Input: part model. Units: mm. Frame: model coordinates. A direction names the side the tool comes from. Coordinates: 2 decimals unless noted, no trailing zeros. Loops run counter-clockwise (first coordinate to the right, second up) from the corner with the lowest first, then second, coordinate; pieces in that order, holes last. Notation, with made-up numbers: (26.5, 51.25) -> (34.5, 51.25) arc R12 cw to (34.5, 66.25) -> close; hole circle Ø4 at (-27.5, 44). An arc over 180 degrees is marked (long way). Answer as a JSON object with one key per item and string values.
Autodesk Inventor part; units mm, degrees
ref_plane "YZ Plane" through (0, 0, 0) normal (1, 0, 0) x (0, 1, 0)
ref_plane "XZ Plane" through (0, 0, 0) normal (0, 1, 0) x (-1, 0, 0)
ref_plane "XY Plane" through (0, 0, 0) normal (0, 0, 1) x (1, 0, 0)
sketch "Sketch1" plane through (0, 0, 0) normal (0, 0, 1) x (1, 0, 0)
  line L0 (-8.8422, 6.5161) -> (13.7638, 6.5161)
  line L1 (13.7638, -16.0899) -> (-8.8422, -16.0899)
  circle A0 centre (2.4608, -4.7869) radius 4.8768
  arc A1 (-8.8422, -9.6637) -> (-8.8422, 0.0899) centre (-8.8422, -4.7869) ccw
  line L2 (-8.8422, -16.0899) -> (-8.8422, -9.6637)
  line L3 (-8.8422, 0.0899) -> (-8.8422, 6.5161)
  arc A2 (13.7638, 0.0899) -> (13.7638, -9.6637) centre (13.7638, -4.7869) ccw
  line L4 (13.7638, 6.5161) -> (13.7638, 0.0899)
  line L5 (13.7638, -9.6637) -> (13.7638, -16.0899)
  dimension "d2" = 22.606
  dimension "d3" = 22.606
  dimension "d4" = 9.7536
  dimension "d5" = 9.7536
extrude "Extrusion1" add sketch "Sketch1" along normal blind 1.397
fillet "Fillet1" radius 3.175 4 edges at (-8.8422, 6.5161, 0.6985) (13.7638, 6.5161, 0.6985) (13.7638, -16.0899, 0.6985) (-8.8422, -16.0899, 0.6985)
sketch "Sketch2" plane through (0, 0, 1.397) normal (0, 0, 1) x (1, 0, 0)
  line L0 (-8.8422, 3.3411) -> (-8.8422, 0.0899)
  circle A0 centre (-6.5606, 4.3162) radius 1.397
  line L1 (10.5888, 6.5161) -> (-5.6672, 6.5161)
  arc A1 (-8.8422, -9.6637) -> (-8.8422, 0.0899) centre (-8.8422, -4.7869) ccw
  arc A2 (13.7638, 0.0899) -> (13.7638, -9.6637) centre (13.7638, -4.7869) ccw
  circle A3 centre (-6.5606, -13.89) radius 1.397
  line L2 (-5.6672, -16.0899) -> (10.5888, -16.0899)
  circle A4 centre (11.4822, 4.3162) radius 1.397
  circle A5 centre (11.4822, -13.89) radius 1.397
  point P0 (0, 0)
  dimension "d9" = 2.794
extrude "Extrusion2" cut sketch "Sketch2" against normal blind 1.397
sketch "Sketch3" plane through (0, 0, 1.397) normal (0, 0, 1) x (1, 0, 0)
  line L0 (2.4608, -16.0899) -> (2.4608, -9.6637)
  circle A0 centre (2.4608, -4.7869) radius 4.8768
  line L1 (2.4608, -16.0899) -> (0.1367, -16.0899)
  line L2 (-3.0383, -16.0899) -> (7.9599, -16.0899)
  line L3 (2.4608, -16.0899) -> (7.9599, -16.0899)
  line L4 (2.4608, -16.0899) -> (7.9599, -16.0899)
  line L5 (10.5888, -16.0899) -> (-5.6672, -16.0899)
  line L6 (7.9599, -17.9949) -> (7.9599, -16.0899)
  line L7 (-3.0383, -17.9949) -> (-3.0383, -16.0899)
  line L8 (-3.0383, -17.9949) -> (-3.0383, -19.8999)
  line L9 (-3.0383, -19.8999) -> (7.9599, -19.8999)
  line L10 (7.9599, -19.8999) -> (7.9599, -17.9949)
  point P0 (0, 0)
  point P1 (-5.6672, -16.0899)
  dimension "d12" = 5.4991
  dimension "d13" = 5.4991
  dimension "d14" = 1.905
  dimension "d16" = 1.905
extrude "Extrusion3" add sketch "Sketch3" against normal blind 1.397 contours L2 L6 L10 L9 L8 L7 L1
fillet "Fillet2" radius 1.27 2 edges at (7.9599, -16.0899, 0.6985) (-3.0383, -16.0899, 0.6985)
sketch "Sketch4" plane through (-3.0383, -19.8999, 1.397) normal (0, -1, 0) x (1, 0, 0)
  line L0 (10.9982, -1.397) -> (0, -1.397)
  line L1 (10.9982, -1.397) -> (10.9982, -3.4544)
  line L2 (10.9982, -3.4544) -> (0, -3.4544)
  line L3 (0, -3.4544) -> (0, -1.397)
  point P0 (3.0383, -1.397)
  dimension "d20" = 2.0574
extrude "Extrusion4" add sketch "Sketch4" along normal blind 1.397
sketch "Sketch5" plane through (-3.0383, -19.8999, 1.397) normal (0, 1, 0) x (1, 0, 0)
  line L0 (10.9982, 3.4544) -> (10.9982, 1.397)
  line L1 (10.9982, 3.4544) -> (-5.5499, 3.4544)
  line L2 (-5.5499, 3.4544) -> (-5.5499, 14.4526)
  line L3 (-5.5499, 14.4526) -> (16.4973, 14.4526)
  line L4 (10.9982, 1.397) -> (0, 1.397)
  line L5 (0, 3.4544) -> (10.9982, 3.4544)
  line L6 (0, 3.4544) -> (10.9982, 3.4544)
  line L7 (16.4973, 14.4526) -> (16.4973, 3.4544)
  line L8 (16.4973, 3.4544) -> (10.9982, 3.4544)
  point P0 (5.4991, 3.4544)
  point P1 (5.4991, 3.4544)
  dimension "d25" = 22.0472
  dimension "d38" = 10.9982
extrude "Extrusion5" add sketch "Sketch5" against normal blind 1.397
fillet "Fillet3" radius 1.27 2 edges at (-3.0383, -20.5984, -2.0574) (7.9599, -20.5984, -2.0574)
fillet "Fillet4" radius 0.508 4 edges at (-8.5882, -20.5984, -2.0574) (-8.5882, -20.5984, -13.0556) (13.459, -20.5984, -2.0574) (13.459, -20.5984, -13.0556)
sketch "Sketch8" plane through (-3.0383, -19.8999, 0) normal (0, 0, 1) x (1, 0, 0)
  line L0 (0, 0) -> (0, -1.397)
  line L1 (0, -1.397) -> (0, 0)
  line L2 (10.9982, 0) -> (10.9982, -1.397)
  line L3 (0, 0) -> (10.9982, 0)
  line L4 (10.9982, 0) -> (10.9982, -1.397)
  line L5 (10.9982, -1.397) -> (0, -1.397)
  point P0 (3.0383, 19.8999)
extrude "Extrusion8" add sketch "Sketch8" along normal blind 1.397
fillet "Fillet5" radius 1.524 1 edges at (2.4608, -21.2969, 1.397)
sketch "Sketch11" plane through (-3.0383, -19.8999, 1.397) normal (0, 1, 0) x (1, 0, 0)
  line L0 (-5.0419, 14.4526) -> (15.9893, 14.4526)
  line L1 (-2.6289, 1.397) -> (13.6271, 1.397)
  line L2 (16.4973, 13.9446) -> (16.4973, 3.9624)
  line L3 (-5.5499, 13.9446) -> (-5.5499, 3.9624)
  circle A0 centre (13.6271, 11.5283) radius 1.5113
  line L4 (6.7183, 3.3528) -> (6.7183, 11.811)
  line L5 (4.2291, 11.811) -> (4.2291, 3.3528)
  arc A1 (4.2291, 3.3528) -> (6.7183, 3.3528) centre (5.4737, 3.3528) ccw
  arc A2 (6.7183, 11.811) -> (4.2291, 11.811) centre (5.4737, 11.811) ccw
  circle A3 centre (13.6271, 6.3787) radius 1.5113
  line L6 (0, 1.524) -> (10.9982, 1.524)
  circle A4 centre (-2.6681, 11.4963) radius 1.5113
  circle A5 centre (-2.6479, 6.3467) radius 1.5113
  point P0 (5.4737, 7.5819)
  dimension "d43" = 3.0226
  dimension "d47" = 2.8702
  dimension "d50" = 2.6416
  dimension "d51" = 1.9558
extrude "Extrusion10" cut sketch "Sketch11" against normal through all
properties part number "mcdave_mount"
1. Mould query, pull axis Y, two halves, no side actions, for faces 1 (the face through (12.86, 5.56, 0.71)), 2 (the face through (5.08, -8.9, 0.69)), 3 (the face through (-6, -21, -2.057)). Classes: pulls with the +Y half, pulls with the -Y half, needs draft (parallel to the pull), parting line crosses it, or undercut.
Reply:
{"face 1": "pulls with the +Y half", "face 2": "undercut", "face 3": "needs draft"}
2. Section query A-A (z = -8.25). Return loops of the section in (x, y), plus the area to 3 significant figures.
Reply:
{"outline": "(-8.59, -21.3) -> (1.19, -21.3) -> (1.19, -19.9) -> (-8.59, -19.9) -> close; (3.68, -21.3) -> (13.46, -21.3) -> (13.46, -19.9) -> (3.68, -19.9) -> close", "area": "27.3 mm2"}
3. Section query C-C (y = -5.25). Return loops of the section in (x, z).
Reply:
{"outline": "(-3.99, 0) -> (-2.39, 0) -> (-2.39, 1.4) -> (-3.99, 1.4) -> close; (7.32, 0) -> (8.91, 0) -> (8.91, 1.4) -> (7.32, 1.4) -> close"}
4. Section query D-D (x = 11). Return loops of the section in (y, z), plus the area to 3 significant figures.
Reply:
{"outline": "(-21.3, -13.06) -> (-19.9, -13.06) -> (-19.9, -11.59) -> (-21.3, -11.59) -> close; (-21.3, -8.68) -> (-19.9, -8.68) -> (-19.9, -6.44) -> (-21.3, -6.44) -> close; (-21.3, -3.53) -> (-19.9, -3.53) -> (-19.9, -2.06) -> (-21.3, -2.06) -> close; (-16.06, 0) -> (-15.2, 0) -> (-15.2, 1.4) -> (-16.06, 1.4) -> close; (-12.58, 0) -> (-8.8, 0) -> (-8.8, 1.4) -> (-12.58, 1.4) -> close; (-0.77, 0) -> (3.01, 0) -> (3.01, 1.4) -> (-0.77, 1.4) -> close; (5.63, 0) -> (6.49, 0) -> (6.49, 1.4) -> (5.63, 1.4) -> close", "area": "20.2 mm2"}
5. Line query: line 1 along Z through (x, y) = (1.5, -12); line 2 along Y through (x, z) = (9.25, -11.25); line 3 along Y through (x, z) = (5.25, 0.25). Output: solid intervals per line, ascending.
Reply:
{"line 1": "z = 0 to 1.4", "line 2": "y = -21.3 to -19.9", "line 3": "y = -21.25 to -8.79, -0.79 to 6.52"}
6. Pin query (flat end, axial travel): P1, Ø4, axis at x = -5.71, z = -10.1, coming from the +Y side; P2, Ø1.5, axis at y = -20.5, z = -6, coming from the -X side; P3, Ø2.5, axis at x = -6.56, y = 4.32, coming from the +Z side; P4, Ø4, axis at x = -6, y = 0.5, coming from the -Z side. Return the tip coordinate at first contact, or that it passes through.
Reply:
{"P1": "stops at y = -19.9", "P2": "stops at x = -8.59", "P3": "passes through", "P4": "stops at z = 0"}
7. Section query B-B (x = 5.25). Return loops of the section in (y, z), plus the area to 3 significant figures.
Reply:
{"outline": "(-21.3, -13.06) -> (-19.9, -13.06) -> (-19.9, 0) -> (-8.79, 0) -> (-8.79, 1.4) -> (-19.77, 1.4) arc R1.52 ccw to (-21.3, -0.13) -> close; (-0.79, 0) -> (6.52, 0) -> (6.52, 1.4) -> (-0.79, 1.4) -> close", "area": "45.4 mm2"}
8. Access query for faces 4 (the face through (3.68, -21, -6)), 5 (the face through (2, 6.516, 1)). Directions: +Z, -Z, +X, -X, +Y, -Y. A direction counts if a zero-diameter tool reaches every point of the face in a straight line with its end or side. Return the directions, or none.
Reply:
{"face 4": "+Y, -Y", "face 5": "+Z, -Z, +X, -X, +Y"}
